```python
from build123d import *

# Parameters (mm, degrees)
RESSALTO_EXTRUS_O1_DEPTH  = 1.8
ESBO_O2_R                 = 3.65
ESBO_O2_R_2               = 1.245
RESSALTO_EXTRUS_O2_DEPTH  = 4
CORTE_EXTRUS_O1_START     = -2
ESBO_O3_R                 = 2.3
ESBO_O3_R_2               = 1.245
CORTE_EXTRUS_O1_DEPTH     = 2
FURO_COM_FOLGA_DE_00001_D = 0.899999978
FURO_COM_FOLGA_DE_00002_D = 1.000000032


with BuildPart() as part:
    # Esboço1 → Ressalto-extrusão1 (new body)
    with BuildSketch(Plane.XY):
        with BuildLine():
            Line((2, 8.197608696), (3.072718666, 20.297608696))
            ThreePointArc((3.072718666, 20.297608696), (0, 18.617608696), (-3.072718666, 20.297608696))
            Line((-3.072718666, 20.297608696), (-2, 8.197608696))
            ThreePointArc((-2, 8.197608696), (0, 6.36707334), (2, 8.197608696))
        make_face()
    extrude(amount=RESSALTO_EXTRUS_O1_DEPTH)

    # Esboço2 → Ressalto-extrusão2 (add)
    with BuildSketch(Plane(origin=(0, 0, 0), x_dir=(-1, 0, 0), z_dir=(0, 0, -1))):
        with Locations((0, 22.267608696)):
            Circle(ESBO_O2_R)
        with Locations((0, 22.267608696)):
            Circle(ESBO_O2_R_2, mode=Mode.SUBTRACT)
    extrude(amount=-RESSALTO_EXTRUS_O2_DEPTH)

    # Esboço3 → Corte-extrusão1 (cut)
    with BuildSketch(Plane.XY.offset(4).offset(CORTE_EXTRUS_O1_START)):
        with Locations((0, 22.267608696)):
            Circle(ESBO_O3_R)
        with Locations(Location((0, 22.267608696, 0), (0, 0, 180))):
            Circle(ESBO_O3_R_2, mode=Mode.SUBTRACT)
    extrude(amount=CORTE_EXTRUS_O1_DEPTH, mode=Mode.SUBTRACT)

    # Furo com folga de #00001 (through all)
    with Locations(Plane.XY.offset(1.8)):
        with Locations((0, 8.14707334)):
            Hole(FURO_COM_FOLGA_DE_00001_D / 2)

    # Furo com folga de #00002 (through all)
    with Locations(Plane.XY.offset(1.8)):
        with Locations((0, 8.14707334), (0, 9.807341018), (0, 11.467608696), (0, 13.127876373), (0, 14.788144051), (0, 16.448411729)):
            Hole(FURO_COM_FOLGA_DE_00002_D / 2)


solid = part.part
```
CAD build for the part. Positions are in the model's coordinates, mm. A direction names the side the tool comes from. Round coordinates to 2 decimals unless told otherwise and drop trailing zeros. Loops run counter-clockwise (first coordinate to the right, second up) from the corner with the lowest first, then second, coordinate; pieces in that order, holes last. Notation, with made-up numbers: M 52,31 L 64,31 A20 cw 64,40 Z; hole C -29.5,-40 d5. An arc over 180 degrees is marked long. Return JSON: item names as keys, results as strings. Group by question number.
(1) Saw through at A-A, the plane z = 0.35. List the corners of the cut face in (x, y) (3 decimals), and give its area (3 significant figures).
(2) Wall check: probe 1 along Y at (x, z) = (0, 3.5); probe 2 along Z at (x, y) = (2, 15.5); probe 3 along X at (y, z) = (13.5, 1.1). Give the ranges that are in metal, low to high. Write a range as [from, to].
(3) Tool access for faces 1 (the cylindrical face through (-1.962, 25.345, 1.972)), 2 (the cylindrical face through (0.1, 14.3, 0.9)): list every direction of +Z, -Z, +X, -X, +Y, -Y with a clear straight run to the whole face (end or side of a thin tool).
(4) Saw through at B-B, the plane x = 0. Give the number of separate pieces and of enclosed holes in the cut face, and give its area (3 significant figures).
(5) Saw through at C-C, the plane x = 2.75. List the corners of the cut face in (y, z).
(6) Drop flat-ended pins along their axis: P1, Ø0.9, axis at x = 0, y = 8.15, coming from the +Z side; P2, Ø2, axis at y = 13, z = 0.5, coming from the -X side. Give the stop position or say it passes through.
(7) Saw through at D-D, the plane z = 3.15. List the corners of the cut face in (x, y).
Answer list:
{
 "1": {"outline": "M -3.073,20.298 L -2,8.198 A2.008 ccw 2,8.198 L 3.073,20.298 A3.65 ccw long Z; hole C 0,22.268 d2.49; hole C 0,8.147 d1; hole C 0,9.807 d1; hole C 0,11.468 d1; hole C 0,13.128 d1; hole C 0,14.788 d1; hole C 0,16.448 d1", "area": "92.0 mm2"},
 "2": {"probe 1": "[18.62, 19.97], [24.57, 25.92]", "probe 2": "[0, 1.8]", "probe 3": "[-2.47, -0.33], [0.33, 2.47]"},
 "3": {"face 1": "+Z", "face 2": "+Z, -Z"},
 "4": {"separate pieces": "8", "enclosed holes": "0", "area": "26.3 mm2"},
 "5": {"outline": "M 16.66,0 L 24.67,0 L 24.67,4 L 19.87,4 L 19.87,1.8 L 16.66,1.8 Z"},
 "6": {"P1": "through", "P2": "x = -2.51"},
 "7": {"outline": "C 0,22.27 d7.3; hole C 0,22.27 d4.6"}
}
